from build123d import *

# Parameters (mm, degrees)
F0_W           = 12
F0_H           = 50
F0_R           = 2
F0_W_2         = 0.5
F0_W_3         = 10
F1_DEPTH       = 5
F2_DEPTH       = 8.5
F3_SIZE2       = 8
F3_SIZE        = 4.5
F4_SIZE2       = 8
F4_SIZE        = 4.5
F5_D           = 4
F5_CSINK_D     = 8
F5_CSINK_ANGLE = 90
F6_R           = 0.5


with BuildPart() as f1:
    # F0 (on Front) → F1 (new body)
    with BuildSketch(Plane.XZ):
        Rectangle(F0_W, F0_H)
        with Locations((0, -15)):
            Circle(F0_R, mode=Mode.SUBTRACT)
        with Locations((0, 15)):
            Circle(F0_R, mode=Mode.SUBTRACT)
        with Locations((6.25, 0)):
            Rectangle(F0_W_2, F0_H)
        with Locations((-6.25, 0)):
            Rectangle(F0_W_2, F0_H)
        with Locations((11.5, 0)):
            Rectangle(F0_W_3, F0_H)
        with Locations((-11.5, 0)):
            Rectangle(F0_W_3, F0_H)
    extrude(amount=-F1_DEPTH)

    # F0 (on Front) → F2 (join)
    with BuildSketch(Plane.XZ):
        with Locations((-11.5, 0)):
            Rectangle(F0_W_3, F0_H)
        with Locations((11.5, 0)):
            Rectangle(F0_W_3, F0_H)
    extrude(amount=-F2_DEPTH)

    # F3
    f3_edges = [f1.edges().sort_by_distance(p)[0] for p in [
        (-16.5, 8.5, 0),
    ]]
    f3_side = f1.faces().sort_by_distance((-16.5, 4.25, 0))[0]
    chamfer(f3_edges, length=F3_SIZE, length2=F3_SIZE2, reference=f3_side)

    # F4
    f4_edges = [f1.edges().sort_by_distance(p)[0] for p in [
        (16.5, 8.5, 0),
    ]]
    f4_side = f1.faces().sort_by_distance((16.5, 4.25, 0))[0]
    chamfer(f4_edges, length=F4_SIZE, length2=F4_SIZE2, reference=f4_side)

    # F5 (through all)
    with Locations(Plane.XZ):
        with Locations((0, 15), (0, -15)):
            CounterSinkHole(F5_D / 2, F5_CSINK_D / 2, counter_sink_angle=F5_CSINK_ANGLE)

    # F6
    f6_edges = [f1.edges().sort_by_distance(p)[0] for p in [
        (12.5, 6.25, -25),
        (16.5, 4, 0),
        (8.5, 8.5, 0),
        (12.5, 6.25, 25),
        (7.5, 8.5, -25),
        (6.5, 8.5, 0),
        (7.5, 8.5, 25),
        (-7.5, 8.5, -25),
        (-8.5, 8.5, 0),
        (-6.5, 8.5, 0),
        (-7.5, 8.5, 25),
        (-12.5, 6.25, 25),
        (-16.5, 4, 0),
        (-12.5, 6.25, -25),
        (-2, 5, -15),
        (-2, 5, 15),
        (0, 5, -25),
        (6.5, 6.75, -25),
        (-6.5, 6.75, -25),
        (-16.5, 2, -25),
        (16.5, 2, -25),
        (16.5, 2, 25),
        (6.5, 6.75, 25),
        (0, 5, 25),
        (-6.5, 6.75, 25),
        (-16.5, 2, 25),
    ]]
    fillet(f6_edges, radius=F6_R)


solid = f1.part
Can you work these out from the model? Positions are in its coordinate system, mm. A direction names the side the tool comes from. Give positions to 0.01 mm unless a question says otherwise; leave off trailing zeros. Order: outer loops, then holes, each group sorted by start corner. A loop starts at its lowest first (then second) coordinate and runs counter-clockwise, first axis right, second up. Notation, with made-up numbers: M 55,26 L 85,26 A11 ccw 85,43 Z; hole C -2,-19.5 d2. An arc over 180 degrees is marked long. One line per question, with ' | ' between items.
Item 1: I'm going to push flat-ended pins straight in: pin 1 Ø6.5 at (x, z) = (0, 15) entering from -Y; pin 2 Ø10.5 at (x, z) = (3, 0) entering from +Y; pin 3 Ø3.5 at (y, z) = (7, -5.5) entering from +X; pin 4 Ø2 at (y, z) = (5.5, 16.5) entering from -X. Where does each tip first touch, or does it pass through?
Answer block:
pin 1: stops at y = 0.75 | pin 2: stops at y = 8.5 | pin 3: stops at x = 14.28 | pin 4: stops at x = -15.61
Item 2: Suppose I cut it at D-D, the plane x = -1. Give the number of separate pieces and of enclosed holes in the cut face, then the cut area to 3 significant figures.
Answer block:
separate pieces: 3 | enclosed holes: 0 | area: 206 mm2
Item 3: Suppose I cut it at C-C, the plane z = 4. Write out the boundary of the cut face in (x, y), then the cut area to 3 significant figures.
Answer block:
outline: M -16.5,0 L 16.5,0 L 16.5,3.71 A0.5 ccw 16.25,4.14 L 8.61,8.44 A0.5 ccw 8.37,8.5 L 7,8.5 A0.5 ccw 6.5,8 L 6.5,5 L -6.5,5 L -6.5,8 A0.5 ccw -7,8.5 L -8.37,8.5 A0.5 ccw -8.61,8.44 L -16.25,4.14 A0.5 ccw -16.5,3.71 Z | area: 199 mm2
Item 4: For faces 4 (the face through (6.5, 6, 0)), 5 (the face through (-12.376, 6.32, -0.343)), which set-ups out of +Z, -Z, +X, -X, +Y, -Y let a thin tool reach every point of the face, with its end or its side?
Answer block:
face 4: +Z, -Z, +Y | face 5: +Z, -Z, -X, +Y
Item 5: We'd pull the mould along X, two halves only. Please class faces 1 (the face through (0, 3, -25)), 2 (the face through (12.3, 6.19, -24.86)), 3 (the face through (0.923, 3.233, -16.774)): released by +X, released by -X, zero draft, split by the parting line, or undercut.
Answer block:
face 1: zero draft | face 2: released by +X | face 3: undercut
Item 6: Suppose I cut it at B-B, the plane y = 0.75. Write out the boundary of the cut face in (x, z).
Answer block:
outline: M -16.5,-24.5 A0.5 ccw -16,-25 L 16,-25 A0.5 ccw 16.5,-24.5 L 16.5,24.5 A0.5 ccw 16,25 L -16,25 A0.5 ccw -16.5,24.5 Z; hole C 0,-15 d6.5; hole C 0,15 d6.5
Item 7: Suppose I cut it at A-A, the plane z = 15. Write out the boundary of the cut face in (x, y), then the cut area to 3 significant figures.
Answer block:
outline: M -16.5,0 L -4,0 L -2,2 L -2,4.5 A0.5 ccw -2.5,5 L -6.5,5 L -6.5,8 A0.5 ccw -7,8.5 L -8.37,8.5 A0.5 ccw -8.61,8.44 L -16.25,4.14 A0.5 ccw -16.5,3.71 Z; M 2,2 L 4,0 L 16.5,0 L 16.5,3.71 A0.5 ccw 16.25,4.14 L 8.61,8.44 A0.5 ccw 8.37,8.5 L 7,8.5 A0.5 ccw 6.5,8 L 6.5,5 L 2.5,5 A0.5 ccw 2,4.5 Z | area: 175 mm2
Item 8: Please list where these lines run through material, in increasing order: L1, parallel to Z at x = 0, y = 3.35; L2, parallel to X at y = 6.25, z = -13.5; L3, parallel to Z at x = 1.5, y = 3.5.
Answer block:
L1: z = -25 to -17, -13 to 13, 17 to 25 | L2: x = -12.5 to -6.5, 6.5 to 12.5 | L3: z = -25 to -16.32, -13.68 to 13.68, 16.32 to 25
